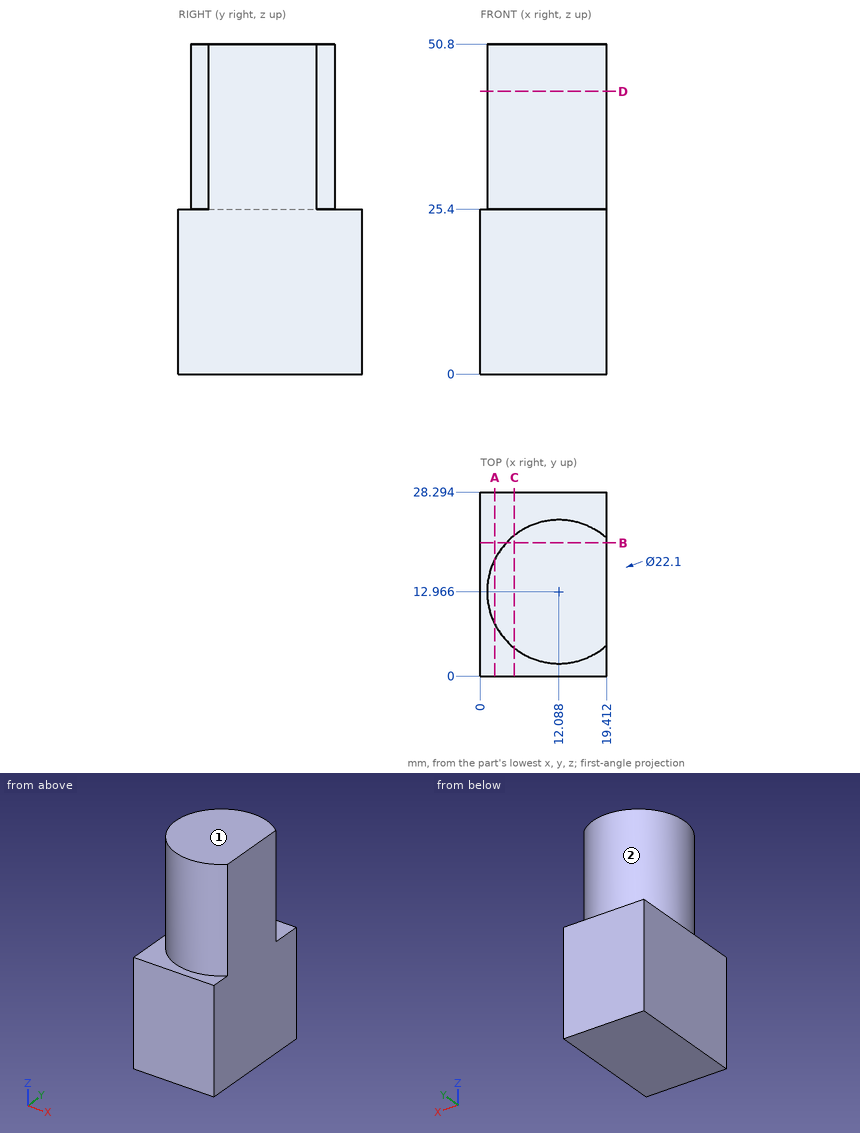
Geometry: see drawing. Coordinates: mm, zero at the bounding-box minimum. A direction names the side the tool comes from. Coordinates: 2 decimals unless noted, no trailing zeros. Order: outer loops, then holes, each group sorted by start corner. A loop starts at its lowest first (then second) coordinate and runs counter-clockwise, first axis right, second up. Notation, with made-up numbers: (-3, -10) - (19, -10) arc R26 ccw to (19, 17) - close; hole circle Ø5 at (7, 54). An arc over 180 degrees is marked (long way). Use one line per item in the form item = value.
1) Ray query, L1, parallel to Z at x = 16.75, y = 2.75; L2, parallel to Y at x = 4.5, z = 42; L3, parallel to Y at x = 17.5, z = 27. Return the intervals inside material, ascending.
Solutions:
L1 = 0 to 25.4
L2 = 4.93 to 21
L3 = 3.33 to 22.6
2) Pin query (flat end, axial travel): pin 1 (5 mm diameter, centred on x = 2, z = 30.5, fed in from +Y); pin 2 (4 mm diameter, centred on x = 2.5, z = 32.5, fed in from -Y); pin 3 (5 mm diameter, centred on y = 16.5, z = 33.5, fed in from -X). Return the tip coordinate at first contact, or that it passes through.
Solutions:
pin_1 = 21
pin_2 = 4.93
pin_3 = 1.09
3) Section D-D (z = 43.5). Return loops of the section in (x, y), then the cut area to 3 significant figures.
Solutions:
outline = (19.41, 4.69) - (19.41, 21.24) arc R11.05 ccw (long way) to start
area = 341 mm^2
4) Section A-A (x = 2.25). Return loops of the section in (y, z) (1 decimal).
Solutions:
outline = (0, 0) - (28.3, 0) - (28.3, 25.4) - (18, 25.4) - (18, 50.8) - (7.9, 50.8) - (7.9, 25.4) - (0, 25.4) - close
5) Set-up query: the marked faces 1 and 2. Return all of +Z, -Z, +X, -X, +Y, -Y with unobstructed straight access to the full face (end or side cutting, diameter ignored); none if empty.
Solutions:
face_1 = +Z, +X, -X, +Y, -Y
face_2 = +Z
6) Section C-C (x = 5.25). Return loops of the section in (y, z) (1 decimal).
Solutions:
outline = (0, 0) - (28.3, 0) - (28.3, 25.4) - (21.6, 25.4) - (21.6, 50.8) - (4.3, 50.8) - (4.3, 25.4) - (0, 25.4) - close
7) Section B-B (y = 20.5). Return loops of the section in (x, z).
Solutions:
outline = (0, 0) - (19.41, 0) - (19.41, 50.8) - (4, 50.8) - (4, 25.4) - (0, 25.4) - close
